The model under review builds one solid part; all positions refer to its coordinate system, in mm. A direction names the side the tool comes from. Round coordinates to 2 decimals unless told otherwise and drop trailing zeros. Loops run counter-clockwise (first coordinate to the right, second up) from the corner with the lowest first, then second, coordinate; pieces in that order, holes last. Notation, with made-up numbers: M 80,15 L 88,15 A19 ccw 88,37 Z; hole C 44.25,19 d3. An arc over 180 degrees is marked long. Return JSON: item names as keys, results as strings. Group by question number.
Q1. Clearance check with flat-ended pins moving along their axes: pin 1 Ø1.8 at (x, y) = (-24, 0) entering from -Z; pin 2 Ø0.8 at (x, y) = (-100.5, -3) entering from +Z. State where each tip first meets the part, or that it passes through.
Q2. To check wall thickness, follow line 1 along Z through (x, y) = (21, 2.25); line 2 along Z through (x, y) = (-81, 3); line 3 along Y through (x, z) = (-33, -4.5). State the ranges of each line that lie inside material, in increasing order.
Q3. Draft analysis for pull direction Z (two halves, no side actions). For faces 1 (the face through (2, -2.5, 3)), 2 (the face through (-2, 3.5, -15)), 3 (the face through (2, -1, -14)), state which applies: pulls with the +Z half, pulls with the -Z half, needs draft (parallel to the pull), parting line crosses it, or undercut.
Q4. Consider section A-A (y = 0.5). State the section outline as (x, z) points.
Q5. Consider section B-B (x = -22). State the section outline as (y, z) points, and give its area (3 significant figures).
Q6. For faces 4 (the face through (2, 2.5, 16)), 5 (the face through (-2, 3.5, 15)), 6 (the face through (2, 1, 13)), 7 (the face through (2, 2.5, -16)), list the 3-axis set-ups (+Z, -Z, +X, -X, +Y, -Y) from which the entire face can be reached by the end or side of a thin tool; tool diameter is ignored.
from build123d import *

# Parameters (mm, degrees)
SKETCH1_W           = 225
SKETCH1_H           = 35
BOSS_EXTRUDE1_DEPTH = 3.5
SKETCH2_W           = 3.5
SKETCH2_H           = 6
CUT_EXTRUDE1_DEPTH  = 226
CUT_EXTRUDE2_DEPTH  = 2


with BuildPart() as part:
    # Sketch1 → Boss-Extrude1 (new body, symmetric)
    with BuildSketch(Plane(origin=(0, 0, 0), x_dir=(1, 0, 0), z_dir=(0, 1, 0))):
        Rectangle(SKETCH1_W, SKETCH1_H)
    extrude(amount=BOSS_EXTRUDE1_DEPTH, both=True)

    # Sketch2 → Cut-Extrude1 (cut, through all)
    with BuildSketch(Plane(origin=(112.5, 0, 0), x_dir=(0, 0, -1), z_dir=(1, 0, 0))):
        Polygon((-13, -2.5), (0, -2.5), (13, -2.5), (13, 3.5), (-13, 3.5), align=None)
        with Locations((15.75, -0.5)):
            Rectangle(SKETCH2_W, SKETCH2_H)
        with Locations((-15.75, -0.5)):
            Rectangle(SKETCH2_W, SKETCH2_H)
    extrude(amount=-CUT_EXTRUDE1_DEPTH, mode=Mode.SUBTRACT)

    # Sketch3 → Cut-Extrude2 (cut, through all)
    with BuildSketch(Plane(origin=(0, -2.5, 0), x_dir=(1, 0, 0), z_dir=(0, 1, 0))):
        with BuildLine():
            Line((-4, 2), (4, 2))
            ThreePointArc((4, 2), (6, 0), (4, -2))
            Line((4, -2), (-4, -2))
            ThreePointArc((-4, -2), (-6, 0), (-4, 2))
        make_face()
        with BuildLine():
            Line((16, 2), (24, 2))
            ThreePointArc((24, 2), (26, 0), (24, -2))
            Line((24, -2), (16, -2))
            ThreePointArc((16, -2), (14, 0), (16, 2))
        make_face()
        with BuildLine():
            Line((36, 2), (44, 2))
            ThreePointArc((44, 2), (46, 0), (44, -2))
            Line((44, -2), (36, -2))
            ThreePointArc((36, -2), (34, 0), (36, 2))
        make_face()
        with BuildLine():
            Line((56, 2), (64, 2))
            ThreePointArc((64, 2), (66, 0), (64, -2))
            Line((64, -2), (56, -2))
            ThreePointArc((56, -2), (54, 0), (56, 2))
        make_face()
        with BuildLine():
            Line((76, 2), (84, 2))
            ThreePointArc((84, 2), (86, 0), (84, -2))
            Line((84, -2), (76, -2))
            ThreePointArc((76, -2), (74, 0), (76, 2))
        make_face()
        with BuildLine():
            Line((-24, 2), (-16, 2))
            ThreePointArc((-16, 2), (-14, 0), (-16, -2))
            Line((-16, -2), (-24, -2))
            ThreePointArc((-24, -2), (-26, 0), (-24, 2))
        make_face()
        with BuildLine():
            Line((-44, 2), (-36, 2))
            ThreePointArc((-36, 2), (-34, 0), (-36, -2))
            Line((-36, -2), (-44, -2))
            ThreePointArc((-44, -2), (-46, 0), (-44, 2))
        make_face()
        with BuildLine():
            Line((-64, 2), (-56, 2))
            ThreePointArc((-56, 2), (-54, 0), (-56, -2))
            Line((-56, -2), (-64, -2))
            ThreePointArc((-64, -2), (-66, 0), (-64, 2))
        make_face()
        with BuildLine():
            Line((-84, 2), (-76, 2))
            ThreePointArc((-76, 2), (-74, 0), (-76, -2))
            Line((-76, -2), (-84, -2))
            ThreePointArc((-84, -2), (-86, 0), (-84, 2))
        make_face()
        with BuildLine():
            Line((-104, 2), (-96, 2))
            ThreePointArc((-96, 2), (-94, 0), (-96, -2))
            Line((-96, -2), (-104, -2))
            ThreePointArc((-104, -2), (-106, 0), (-104, 2))
        make_face()
        with BuildLine():
            Line((-124, 2), (-116, 2))
            ThreePointArc((-116, 2), (-114, 0), (-116, -2))
            Line((-116, -2), (-124, -2))
            ThreePointArc((-124, -2), (-126, 0), (-124, 2))
        make_face()
        with BuildLine():
            Line((-144, 2), (-136, 2))
            ThreePointArc((-136, 2), (-134, 0), (-136, -2))
            Line((-136, -2), (-144, -2))
            ThreePointArc((-144, -2), (-146, 0), (-144, 2))
        make_face()
        with BuildLine():
            Line((96, 2), (104, 2))
            ThreePointArc((104, 2), (106, 0), (104, -2))
            Line((104, -2), (96, -2))
            ThreePointArc((96, -2), (94, 0), (96, 2))
        make_face()
        with BuildLine():
            Line((116, 2), (124, 2))
            ThreePointArc((124, 2), (126, 0), (124, -2))
            Line((124, -2), (116, -2))
            ThreePointArc((116, -2), (114, 0), (116, 2))
        make_face()
        with BuildLine():
            Line((136, 2), (144, 2))
            ThreePointArc((144, 2), (146, 0), (144, -2))
            Line((144, -2), (136, -2))
            ThreePointArc((136, -2), (134, 0), (136, 2))
        make_face()
    extrude(amount=-CUT_EXTRUDE2_DEPTH, mode=Mode.SUBTRACT)


solid = part.part
Values:
{
 "1": {"pin 1": "stops at z = -14", "pin 2": "stops at z = 14"},
 "2": {"line 1": "z = -14 to -13, 13 to 14", "line 2": "z = -17.5 to -13, 13 to 17.5", "line 3": "y = -3.5 to -2.5"},
 "3": {"face 1": "undercut", "face 2": "needs draft", "face 3": "pulls with the -Z half"},
 "4": {"outline": "M -112.5,-14 L 112.5,-14 L 112.5,-13 L -112.5,-13 Z; M -112.5,13 L 112.5,13 L 112.5,14 L -112.5,14 Z"},
 "5": {"outline": "M -3.5,-14 L 2.5,-14 L 2.5,-17.5 L 3.5,-17.5 L 3.5,-13 L -2.5,-13 L -2.5,-2 L -3.5,-2 Z; M -3.5,2 L -2.5,2 L -2.5,13 L 3.5,13 L 3.5,17.5 L 2.5,17.5 L 2.5,14 L -3.5,14 Z", "area": "43.0 mm2"},
 "6": {"face 4": "+Z, +X, -X, -Y", "face 5": "+Z, -Z, +X, -X, +Y", "face 6": "+X, -X, +Y", "face 7": "-Z, +X, -X, -Y"}
}
